Input: part model. Units: mm. Frame: model coordinates. Give positions to 0.01 mm unless a question says otherwise; leave off trailing zeros. Write each loop counter-clockwise with the first axis right and the second up, starting at its lowest first coordinate (ties: lowest second). Pieces come first, ordered by that corner, then holes.
```python
from build123d import *

# Parameters (mm, degrees)
SKETCH3_W           = 125
SKETCH3_H           = 205
BOSS_EXTRUDE1_DEPTH = 3
SKETCH4_W           = 15
SKETCH4_H           = 50
SKETCH4_W_2         = 50
SKETCH4_H_2         = 15
CUT_EXTRUDE1_DEPTH  = 6
SKETCH5_W           = 12
SKETCH5_H           = 3
SKETCH5_W_2         = 3
SKETCH5_H_2         = 12
BOSS_EXTRUDE2_DEPTH = 3


with BuildPart() as part:
    # Sketch3 → Boss-Extrude1 (new body)
    with BuildSketch(Plane(origin=(0, 0, 0), x_dir=(1, 0, 0), z_dir=(0, 1, 0))):
        Rectangle(SKETCH3_W, SKETCH3_H)
    extrude(amount=BOSS_EXTRUDE1_DEPTH)

    # Sketch4 → Cut-Extrude1 (cut)
    with BuildSketch(Plane(origin=(0, 3, 0), x_dir=(1, 0, 0), z_dir=(0, 1, 0))):
        with Locations((-40, 40)):
            Rectangle(SKETCH4_W, SKETCH4_H)
        with Locations((40, 40)):
            Rectangle(SKETCH4_W, SKETCH4_H)
        Rectangle(SKETCH4_W_2, SKETCH4_H_2)
        with Locations((-40, -40)):
            Rectangle(SKETCH4_W, SKETCH4_H)
        with Locations((40, -40)):
            Rectangle(SKETCH4_W, SKETCH4_H)
        with Locations((0, 80)):
            Rectangle(SKETCH4_W_2, SKETCH4_H_2)
        with Locations((0, -80)):
            Rectangle(SKETCH4_W_2, SKETCH4_H_2)
    extrude(amount=-CUT_EXTRUDE1_DEPTH, mode=Mode.SUBTRACT)

    # Sketch5 → Boss-Extrude2 (add)
    with BuildSketch(Plane(origin=(0, 3, 0), x_dir=(1, 0, 0), z_dir=(0, 1, 0))):
        with Locations((24, -104)):
            Rectangle(SKETCH5_W, SKETCH5_H)
        with Locations((0, -104)):
            Rectangle(SKETCH5_W, SKETCH5_H)
        with Locations((-64, -84)):
            Rectangle(SKETCH5_W_2, SKETCH5_H_2)
        with Locations((-64, -60)):
            Rectangle(SKETCH5_W_2, SKETCH5_H_2)
        with Locations((-64, -12)):
            Rectangle(SKETCH5_W_2, SKETCH5_H_2)
        with Locations((64, -84)):
            Rectangle(SKETCH5_W_2, SKETCH5_H_2)
        with Locations((64, -36)):
            Rectangle(SKETCH5_W_2, SKETCH5_H_2)
        with Locations((64, -12)):
            Rectangle(SKETCH5_W_2, SKETCH5_H_2)
        with Locations((64, 12)):
            Rectangle(SKETCH5_W_2, SKETCH5_H_2)
        with Locations((64, 36)):
            Rectangle(SKETCH5_W_2, SKETCH5_H_2)
        with Locations((64, 84)):
            Rectangle(SKETCH5_W_2, SKETCH5_H_2)
        with Locations((24, 104)):
            Rectangle(SKETCH5_W, SKETCH5_H)
        with Locations((0, 104)):
            Rectangle(SKETCH5_W, SKETCH5_H)
        with Locations((-24, 104)):
            Rectangle(SKETCH5_W, SKETCH5_H)
        with Locations((-48, 104)):
            Rectangle(SKETCH5_W, SKETCH5_H)
        with Locations((-64, 36)):
            Rectangle(SKETCH5_W_2, SKETCH5_H_2)
        with Locations((-64, 12)):
            Rectangle(SKETCH5_W_2, SKETCH5_H_2)
        with Locations((48, -104)):
            Rectangle(SKETCH5_W, SKETCH5_H)
        with Locations((-24, -104)):
            Rectangle(SKETCH5_W, SKETCH5_H)
        with Locations((-48, -104)):
            Rectangle(SKETCH5_W, SKETCH5_H)
        with Locations((-64, -36)):
            Rectangle(SKETCH5_W_2, SKETCH5_H_2)
        with Locations((64, -60)):
            Rectangle(SKETCH5_W_2, SKETCH5_H_2)
        with Locations((64, 60)):
            Rectangle(SKETCH5_W_2, SKETCH5_H_2)
        with Locations((48, 104)):
            Rectangle(SKETCH5_W, SKETCH5_H)
        with Locations((-64, 84)):
            Rectangle(SKETCH5_W_2, SKETCH5_H_2)
        with Locations((-64, 60)):
            Rectangle(SKETCH5_W_2, SKETCH5_H_2)
    extrude(amount=-BOSS_EXTRUDE2_DEPTH)


solid = part.part
```
Q1. Section A-A, the plane x = -39. Return the cut outline in (y, z), then the cut area to 3 significant figures.
Q2. Material intervals for line 1 along Z through (x, y) = (-8, 1.2); line 2 along X through (y, z) = (2.5, 31); line 3 along X through (y, z) = (2.45, 49), sorted ascending.
Q3. Section C-C, the plane z = -61.5. Return the cut outline in (x, y), then the cut area to 3 significant figures.
Q4. Pin query (flat end, axial travel): pin 1 (1.5 mm diameter, centred on y = 2.5, z = -24.5, fed in from +X); pin 2 (0.9 mm diameter, centred on y = 2, z = 104, fed in from +X); pin 3 (1.5 mm diameter, centred on y = 2, z = 104.5, fed in from -X). Return the tip coordinate at first contact, or that it passes through.
Q5. Section B-B, the plane x = -3. Return the cut outline in (y, z).
Q6. Section D-D, the plane y = 1.2. Give the number of separate pieces and of enclosed holes in the cut face, then the cut area to 3 significant figures.
Solutions:
1. outline: (0, -102.5) - (3, -102.5) - (3, -65) - (0, -65) - close; (0, -15) - (3, -15) - (3, 15) - (0, 15) - close; (0, 65) - (3, 65) - (3, 102.5) - (0, 102.5) - close
1. area: 315 mm2
2. line 1: z = -102.5 to -87.5, -72.5 to -7.5, 7.5 to 72.5, 87.5 to 102.5
2. line 2: x = -65.5 to -47.5, -32.5 to 32.5, 47.5 to 65.5
2. line 3: x = -62.5 to -47.5, -32.5 to 32.5, 47.5 to 62.5
3. outline: (-65.5, 0) - (-47.5, 0) - (-47.5, 3) - (-65.5, 3) - close; (-32.5, 0) - (32.5, 0) - (32.5, 3) - (-32.5, 3) - close; (47.5, 0) - (65.5, 0) - (65.5, 3) - (47.5, 3) - close
3. area: 303 mm2
4. pin 1: stops at x = 62.5
4. pin 2: stops at x = 54
4. pin 3: stops at x = -54
5. outline: (0, -105.5) - (3, -105.5) - (3, -87.5) - (0, -87.5) - close; (0, -72.5) - (3, -72.5) - (3, -7.5) - (0, -7.5) - close; (0, 7.5) - (3, 7.5) - (3, 72.5) - (0, 72.5) - close; (0, 87.5) - (3, 87.5) - (3, 105.5) - (0, 105.5) - close
6. separate pieces: 1
6. enclosed holes: 7
6. area: 21,300 mm2
